from build123d import *

# Parameters (mm, degrees)
F0_W     = 49
F0_H     = 82
F0_W_2   = 40
F0_H_2   = 74
F0_W_3   = 7
F0_H_3   = 12
F0_H_4   = 11.5
F1_DEPTH = 4
F2_T     = -1
F4_D     = 3


# Not quite as in the source:
# - a feature names something its author has since deleted; it is built from what else it names


with BuildPart() as f1:
    # F0 (on Front) → F1 (new body)
    with BuildSketch(Plane.XZ):
        with Locations((33.611113002, 41)):
            Rectangle(F0_W, F0_H)
        with Locations((34.111113002, 41)):
            Rectangle(F0_W_2, F0_H_2, mode=Mode.SUBTRACT)
        with Locations((34.111113002, 41)):
            Rectangle(F0_W_2, F0_H_2)
        with Locations((19.111113002, 11.5)):
            Rectangle(F0_W_3, F0_H_3, mode=Mode.SUBTRACT)
        with Locations((29.111113002, 11.5)):
            Rectangle(F0_W_3, F0_H_3, mode=Mode.SUBTRACT)
        with Locations((19.111113002, 26.5)):
            Rectangle(F0_W_3, F0_H_3, mode=Mode.SUBTRACT)
        with Locations((29.111113002, 26.5)):
            Rectangle(F0_W_3, F0_H_3, mode=Mode.SUBTRACT)
        with Locations((39.111113002, 11.5)):
            Rectangle(F0_W_3, F0_H_3, mode=Mode.SUBTRACT)
        with Locations((49.111113002, 11.5)):
            Rectangle(F0_W_3, F0_H_3, mode=Mode.SUBTRACT)
        with Locations((39.111113002, 26.5)):
            Rectangle(F0_W_3, F0_H_3, mode=Mode.SUBTRACT)
        with Locations((49.111113002, 26.5)):
            Rectangle(F0_W_3, F0_H_3, mode=Mode.SUBTRACT)
        with Locations((19.111113002, 41.5)):
            Rectangle(F0_W_3, F0_H_3, mode=Mode.SUBTRACT)
        with Locations((19.111113002, 56.25)):
            Rectangle(F0_W_3, F0_H_4, mode=Mode.SUBTRACT)
        with Locations((29.111113002, 41.5)):
            Rectangle(F0_W_3, F0_H_3, mode=Mode.SUBTRACT)
        with Locations((29.111113002, 56.25)):
            Rectangle(F0_W_3, F0_H_4, mode=Mode.SUBTRACT)
        with Locations((19.111113002, 71)):
            Rectangle(F0_W_3, F0_H_3, mode=Mode.SUBTRACT)
        with Locations((29.111113002, 71)):
            Rectangle(F0_W_3, F0_H_3, mode=Mode.SUBTRACT)
        with Locations((39.111113002, 41.5)):
            Rectangle(F0_W_3, F0_H_3, mode=Mode.SUBTRACT)
        with Locations((39.111113002, 56.25)):
            Rectangle(F0_W_3, F0_H_4, mode=Mode.SUBTRACT)
        with Locations((49.111113002, 41.5)):
            Rectangle(F0_W_3, F0_H_3, mode=Mode.SUBTRACT)
        with Locations((49.111113002, 56.25)):
            Rectangle(F0_W_3, F0_H_4, mode=Mode.SUBTRACT)
        with Locations((39.111113002, 71)):
            Rectangle(F0_W_3, F0_H_3, mode=Mode.SUBTRACT)
        with Locations((49.111113002, 71)):
            Rectangle(F0_W_3, F0_H_3, mode=Mode.SUBTRACT)
    extrude(amount=F1_DEPTH)

    # F2
    f2_openings = [f1.faces().sort_by_distance(p)[0] for p in [
        (33.256946, -4, 40.840774),
    ]]
    offset(amount=F2_T, openings=f2_openings, kind=Kind.INTERSECTION)

    # F4 (through all)
    with Locations(Plane(origin=(0, 0, 0), x_dir=(1, 0, 0), z_dir=(0, 0, -1))):
        with Locations((11.111113002, 2)):
            Hole(F4_D / 2)


solid = f1.part
Geometry check sheet. Reference: the model listing, model coordinates, mm. A direction names the side the tool comes from. Coordinates: 2 decimals unless noted, no trailing zeros. Use a Markdown table: item, result. Add a question column.
1. Go/stop test with a flat-tipped pin: pin 1 Ø1.5 at (x, y) = (40, -2) entering from -Z. Record where the tip stops, or that it passes through.
2. Material ranges on L1, parallel to Z at x = 32, y = -0.55; L2, parallel to Z at x = 24, y = -2.6; L3, parallel to Y at x = 55, z = 31, recorded low to high.
3. Set-up check for faces 1 (the face through (33.611, -2, 41)), 2 (the face through (19, -2, 77)): record each of +Z, -Z, +X, -X, +Y, -Y from which the full face is reachable in a straight line by a thin tool's end or side.
4. Cross-section at A-A (x = 37). Give the number of separate pieces and of enclosed holes in the cut face, and give its area (3 significant figures).
5. Mould release check, pull along X, two halves, no side actions. Record for faces 3 (the face through (19, -2, 64)), 4 (the face through (15, -4, 56)), 5 (the face through (15.611, -2, 11)): pulls with the +X half, pulls with the -X half, needs draft (parallel to the pull), parting line crosses it, or undercut.
Filled sheet:
| question | item | result |
|---|---|---|
| 1 | pin 1 | z = 0 |
| 2 | L1 | 0 to 5.5, 17.5 to 20.5, 32.5 to 35.5, 47.5 to 50.5, 62 to 65, 77 to 82 |
| 2 | L2 | 0 to 1, 81 to 82 |
| 2 | L3 | -1 to 0 |
| 3 | face 1 | -Y |
| 3 | face 2 | +Y, -Y |
| 4 | separate pieces | 6 |
| 4 | enclosed holes | 0 |
| 4 | area | 58.5 mm2 |
| 5 | face 3 | undercut |
| 5 | face 4 | needs draft |
| 5 | face 5 | undercut |
